Here's the drawing with two shaded views (mm, measured from the low corner). I have some questions. A direction names the side the tool comes from. Give positions to 0.01 mm unless a question says otherwise; leave off trailing zeros. Write each loop counter-clockwise with the first axis right and the second up, starting at its lowest first coordinate (ties: lowest second). Pieces come first, ordered by that corner, then holes. Notation, with made-up numbers: (13, 75) -> (52, 75) arc R28 ccw to (52, 112) -> close; hole circle Ø6 at (-4.75, -10.75). An arc over 180 degrees is marked (long way). One line per item, written item: value.
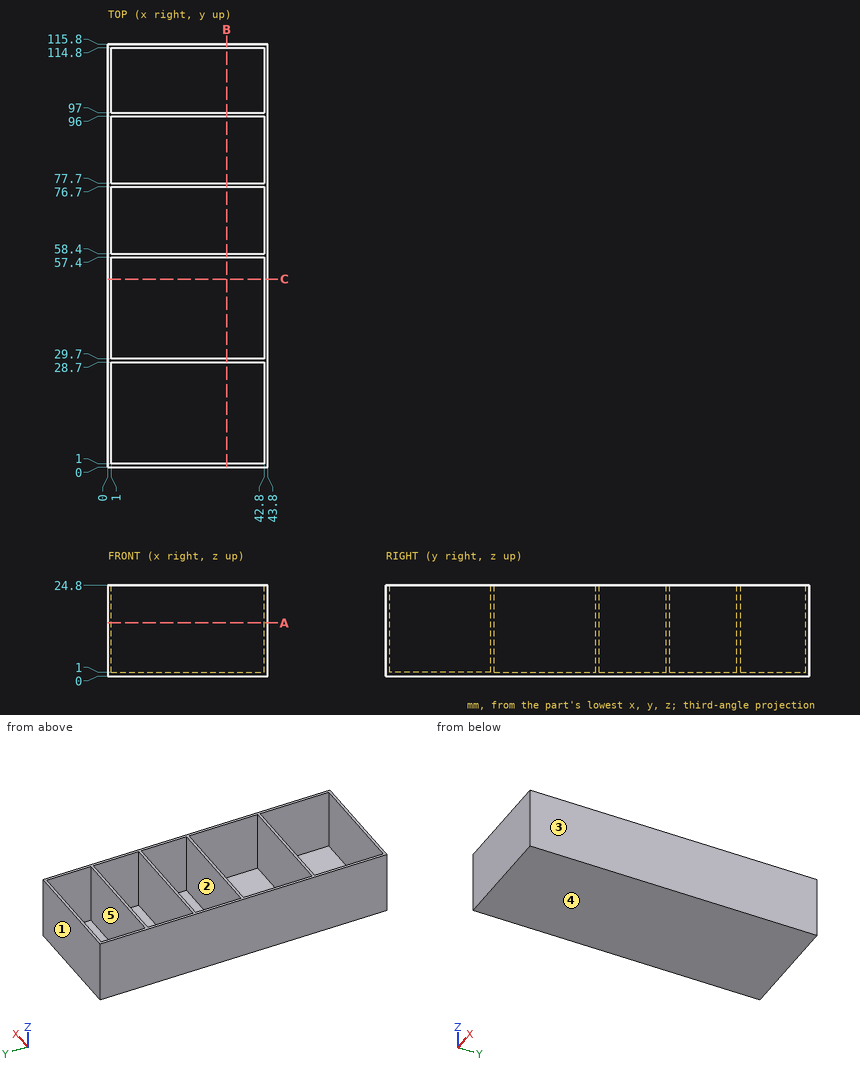
1) We'd pull the mould along Y, two halves only. Please class the marked faces 1, 2 and 3: released by +Y, released by -Y, zero draft, split by the parting line, or undercut.
Answer list:
face 1: released by +Y
face 2: undercut
face 3: zero draft
2) If we section it at C-C (y = 51.5): Write out the boundary of the cut face in (x, z).
Answer list:
outline: (0, 0) -> (43.8, 0) -> (43.8, 24.8) -> (42.8, 24.8) -> (42.8, 1) -> (1, 1) -> (1, 24.8) -> (0, 24.8) -> close
3) If we section it at A-A (z = 14.5): Write out the boundary of the cut face in (x, y).
Answer list:
outline: (0, 0) -> (43.8, 0) -> (43.8, 115.8) -> (0, 115.8) -> close; hole (1, 1) -> (42.8, 1) -> (42.8, 28.7) -> (1, 28.7) -> close; hole (1, 29.7) -> (42.8, 29.7) -> (42.8, 57.4) -> (1, 57.4) -> close; hole (1, 58.4) -> (42.8, 58.4) -> (42.8, 76.7) -> (1, 76.7) -> close; hole (1, 77.7) -> (42.8, 77.7) -> (42.8, 96) -> (1, 96) -> close; hole (1, 97) -> (42.8, 97) -> (42.8, 114.8) -> (1, 114.8) -> close
4) If we section it at B-B (x = 32.5): Write out the boundary of the cut face in (y, z).
Answer list:
outline: (0, 0) -> (115.8, 0) -> (115.8, 24.8) -> (114.8, 24.8) -> (114.8, 1) -> (97, 1) -> (97, 24.8) -> (96, 24.8) -> (96, 1) -> (77.7, 1) -> (77.7, 24.8) -> (76.7, 24.8) -> (76.7, 1) -> (58.4, 1) -> (58.4, 24.8) -> (57.4, 24.8) -> (57.4, 1) -> (29.7, 1) -> (29.7, 24.8) -> (28.7, 24.8) -> (28.7, 1) -> (1, 1) -> (1, 24.8) -> (0, 24.8) -> close
5) I need wall thicknesses on L1, parallel to Y at x = 12.5, z = 18.25; L2, parallel to X at y = 79.5, z = 7.25; L3, parallel to Z at x = 16.5, y = 74. Which ranges of each line are inside material? Lowest first, please.
Answer list:
L1: y = 0 to 1, 28.7 to 29.7, 57.4 to 58.4, 76.7 to 77.7, 96 to 97, 114.8 to 115.8
L2: x = 0 to 1, 42.8 to 43.8
L3: z = 0 to 1
6) Will this pin go through, and if not, where does the flat tip stop? pin 1 (9 mm diameter, centred on x = 28.5, y = 70.5, fed in from +Z).
Answer list:
pin 1: stops at z = 1
7) For the marked faces 4 and 5, which set-ups out of +Z, -Z, +X, -X, +Y, -Y let a thin tool reach every point of the face, with its end or its side?
Answer list:
face 4: -Z, +X, -X, +Y, -Y
face 5: +Z
